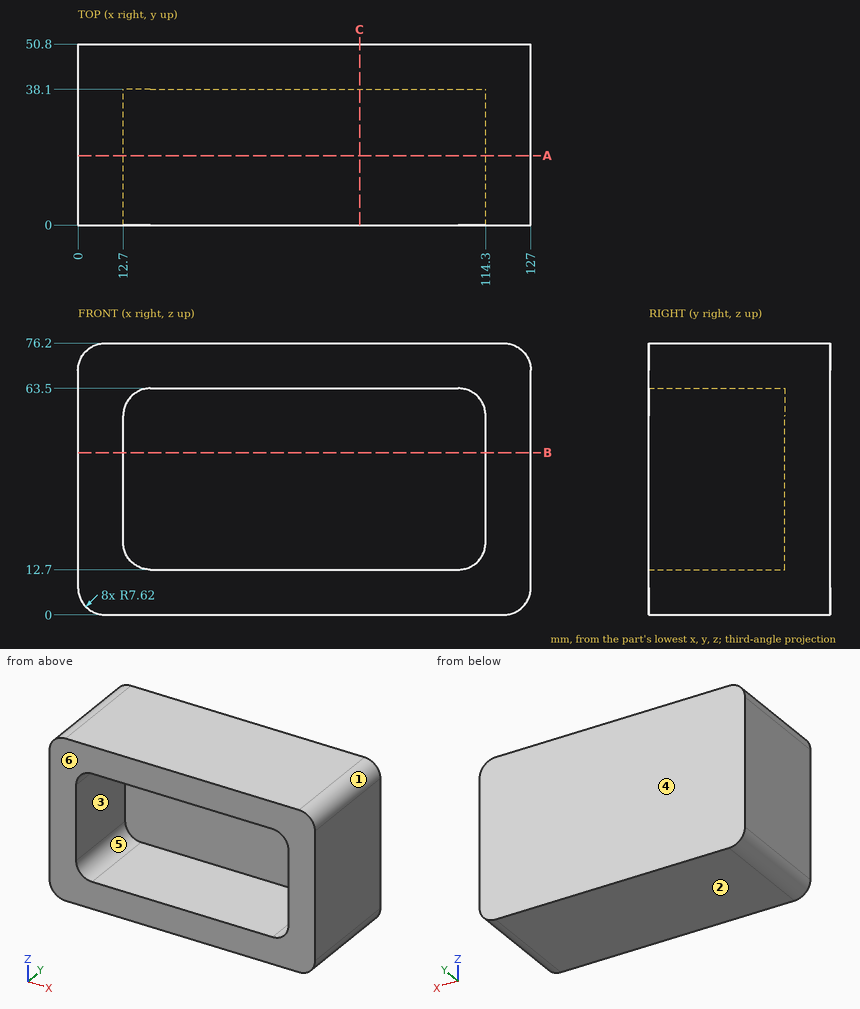
For this review, use the dimensioned drawing (mm, ordinates from the lowest corner) and the shaded views. A direction names the side the tool comes from. Give positions to 0.01 mm unless a question says otherwise; leave off trailing zeros. Order: outer loops, then holes, each group sorted by start corner. A loop starts at its lowest first (then second) coordinate and runs counter-clockwise, first axis right, second up.
1. Tool access review of the marked faces 5 and 6: name each direction out of +Z, -Z, +X, -X, +Y, -Y from which nothing blocks a thin tool from reaching the whole face with its end or side.
Solution:
face 5: -Y
face 6: +Z, -Z, +X, -X, -Y
2. Add section C-C, the plane x = 79. State the section outline as (y, z) points.
Solution:
outline: (0, 0) - (50.8, 0) - (50.8, 76.2) - (0, 76.2) - (0, 63.5) - (38.1, 63.5) - (38.1, 12.7) - (0, 12.7) - close
3. Mouldability with a two-part tool opening along Z and no side actions: class the marked faces 1, 2, 3 and 4 as +Z half, -Z half, draft (parallel to the pull), parting line (faces both ways), or undercut.
Solution:
face 1: +Z half
face 2: -Z half
face 3: undercut
face 4: draft
4. Add section B-B, the plane z = 45.5. State the section outline as (x, y) points, then the cut area to 3 significant figures.
Solution:
outline: (0, 0) - (12.7, 0) - (12.7, 38.1) - (114.3, 38.1) - (114.3, 0) - (127, 0) - (127, 50.8) - (0, 50.8) - close
area: 2,580 mm2
5. Add section A-A, the plane y = 19.5. State the section outline as (x, z) points, then the cut area to 3 significant figures.
Solution:
outline: (0, 7.62) arc R7.62 ccw to (7.62, 0) - (119.38, 0) arc R7.62 ccw to (127, 7.62) - (127, 68.58) arc R7.62 ccw to (119.38, 76.2) - (7.62, 76.2) arc R7.62 ccw to (0, 68.58) - close; hole (12.7, 20.32) arc R7.62 ccw to (20.32, 12.7) - (106.68, 12.7) arc R7.62 ccw to (114.3, 20.32) - (114.3, 55.88) arc R7.62 ccw to (106.68, 63.5) - (20.32, 63.5) arc R7.62 ccw to (12.7, 55.88) - close
area: 4,520 mm2
6. For pin 1 Ø3 at (x, z) = (107, 24) entering from -Y, flat-tipped, find the tip position at first contact; note if it passes through.
Solution:
pin 1: stops at y = 38.1
7. To check wall thickness, follow L1, parallel to X at y = 25.5, z = 51; L2, parallel to Z at x = 47.5, y = 14; L3, parallel to Y at x = 68, z = 40. State the ranges of each line that lie inside material, in increasing order.
Solution:
L1: x = 0 to 12.7, 114.3 to 127
L2: z = 0 to 12.7, 63.5 to 76.2
L3: y = 38.1 to 50.8
